For this review, take the finished solid that the model builds, in its own axes (mm). Face numbers are marked on the shaded views. A direction names the side the tool comes from. Coordinates: 2 decimals unless noted, no trailing zeros. Loops run counter-clockwise (first coordinate to the right, second up) from the corner with the lowest first, then second, coordinate; pieces in that order, holes last. Notation, with made-up numbers: (72, -10) -> (116, -10) arc R21 cw to (116, 4) -> close; hole circle Ø6 at (37.5, 86). An arc over 180 degrees is marked (long way). Answer in a Markdown table with one row per item.
from build123d import *

# Parameters (mm, degrees)
SKETCH_1_R          = 1
EXTRUDE_1_DEPTH     = 2
SKETCH_2_W          = 41
SKETCH_2_H          = 25.9
EXTRUDE_2_DEPTH     = 9.6
CUT_EXTRUDE_1_DEPTH = 49.428323324
CUT_EXTRUDE_2_DEPTH = 0.7
SKETCH_5_R          = 1.25
EXTRUDE_3_DEPTH     = 2
SKETCH_6_R          = 4
EXTRUDE_4_DEPTH     = 4
EXTRUDE_4_TAPER     = 10
SKETCH_7_R          = 2.1
EXTRUDE_5_DEPTH     = 2
SKETCH_8_W          = 12
SKETCH_8_H          = 4.5
CUT_EXTRUDE_3_DEPTH = 0.5
SKETCH_9_W          = 7
SKETCH_9_H          = 4.2
SKETCH_9_W_2        = 6
CUT_EXTRUDE_4_DEPTH = 0.5
SKETCH_12_W         = 3
SKETCH_12_H         = 1
CUT_EXTRUDE_5_DEPTH = 0.5
SKETCH_13_W         = 1.5
SKETCH_13_H         = 1
EXTRUDE_6_DEPTH     = 1


with BuildPart() as part:
    # 草图1 → 凸台-拉伸1 (new body)
    with BuildSketch(Plane(origin=(0, 0, 0), x_dir=(1, 0, 0), z_dir=(0, 1, 0))):
        Polygon((-20.75, 12.95), (20.75, 12.95), (24.7, 9.5), (24.7, -9.5), (20.75, -12.95), (-20.75, -12.95), (-24.7, -9.5), (-24.7, 9.5), align=None)
        with Locations(Location((22.5, 9, 0), (0, 0, 270))):
            Circle(SKETCH_1_R, mode=Mode.SUBTRACT)
        with Locations(Location((22.5, -9, 0), (0, 0, 270))):
            Circle(SKETCH_1_R, mode=Mode.SUBTRACT)
        with Locations(Location((-22.5, -9, 0), (0, 0, 270))):
            Circle(SKETCH_1_R, mode=Mode.SUBTRACT)
        with Locations(Location((-22.5, 9, 0), (0, 0, 270))):
            Circle(SKETCH_1_R, mode=Mode.SUBTRACT)
    extrude(amount=EXTRUDE_1_DEPTH)

    # 草图2 → 凸台-拉伸2 (add)
    with BuildSketch(Plane(origin=(0, 2, 0), x_dir=(1, 0, 0), z_dir=(0, 1, 0))):
        Rectangle(SKETCH_2_W, SKETCH_2_H)
    extrude(amount=EXTRUDE_2_DEPTH)

    # 草图3 → 切除-拉伸1 (cut, through all)
    with BuildSketch(Plane(origin=(20.5, 0, 0), x_dir=(0, 0, -1), z_dir=(1, 0, 0))):
        Polygon((-5.5, 11.6), (-12.95, 10.9), (-12.95, 11.6), align=None)
        Polygon((12.95, 11.6), (5.5, 11.6), (12.95, 10.9), align=None)
    extrude(amount=-CUT_EXTRUDE_1_DEPTH, mode=Mode.SUBTRACT)

    # 草图4 → 切除-拉伸2 (cut)
    with BuildSketch(Plane(origin=(0, 11.6, 0), x_dir=(1, 0, 0), z_dir=(0, 1, 0))):
        Polygon((7.476685986, 12.95), (0, 0), (7.476685986, -12.95), (5.167284909, -12.95), (-2.309401077, 0), (5.167284909, 12.95), align=None)
        Polygon((2.857883832, 12.95), (-1.443375673, 5.5), (-10.840856662, 5.5), (-15.142116168, 12.95), align=None)
        Polygon((-1.443375673, -5.5), (2.857883832, -12.95), (-15.142116168, -12.95), (-10.840856662, -5.5), align=None)
    extrude(amount=-CUT_EXTRUDE_2_DEPTH, mode=Mode.SUBTRACT)

    # 草图5 → 凸台-拉伸3 (add)
    with BuildSketch(Plane.ZY.offset(20.5)):
        with Locations(Location((0, 3.5, 0), (0, 0, 180))):
            Circle(SKETCH_5_R)
        with Locations(Location((4, 3.5, 0), (0, 0, 180))):
            Circle(SKETCH_5_R)
        with Locations(Location((-4, 3.5, 0), (0, 0, 180))):
            Circle(SKETCH_5_R)
    extrude(amount=EXTRUDE_3_DEPTH)

    # 草图6 → 凸台-拉伸4 (add)
    with BuildSketch(Plane(origin=(20.5, 0, 0), x_dir=(0, 0, -1), z_dir=(1, 0, 0))):
        with Locations((0, 6.3)):
            Circle(SKETCH_6_R)
    extrude(amount=EXTRUDE_4_DEPTH, taper=EXTRUDE_4_TAPER)

    # 草图7 → 凸台-拉伸5 (add)
    with BuildSketch(Plane(origin=(24.5, 0, 0), x_dir=(0, 0, -1), z_dir=(1, 0, 0))):
        with Locations((0, 6.3)):
            Circle(SKETCH_7_R)
    extrude(amount=EXTRUDE_5_DEPTH)

    # 草图8 → 切除-拉伸3 (cut)
    with BuildSketch(Plane.ZY.offset(20.5)):
        with Locations((0, 8.25)):
            Rectangle(SKETCH_8_W, SKETCH_8_H)
    extrude(amount=-CUT_EXTRUDE_3_DEPTH, mode=Mode.SUBTRACT)

    # 草图9 → 切除-拉伸4 (cut)
    with BuildSketch(Plane(origin=(20.5, 0, 0), x_dir=(0, 0, -1), z_dir=(1, 0, 0))):
        with Locations((8.25, 8.1)):
            Rectangle(SKETCH_9_W, SKETCH_9_H)
        with Locations((-8.75, 8.1)):
            Rectangle(SKETCH_9_W_2, SKETCH_9_H)
    extrude(amount=-CUT_EXTRUDE_4_DEPTH, mode=Mode.SUBTRACT)

    # 草图12 → 切除-拉伸5 (cut)
    with BuildSketch(Plane.XY.offset(12.95)):
        with Locations((-0.5, 6.5)):
            Rectangle(SKETCH_12_W, SKETCH_12_H)
    extrude(amount=-CUT_EXTRUDE_5_DEPTH, mode=Mode.SUBTRACT)

    # 草图13 → 凸台-拉伸6 (add)
    with BuildSketch(Plane.XY.offset(12.45)):
        with Locations((0.25, 6.5)):
            Rectangle(SKETCH_13_W, SKETCH_13_H)
    extrude(amount=EXTRUDE_6_DEPTH)


solid = part.part
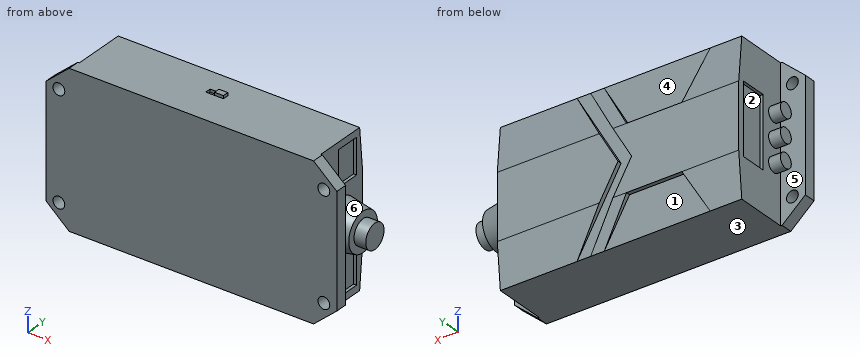
Item 1: For the marked faces 1, 2 and 3, list the 3-axis set-ups (+Z, -Z, +X, -X, +Y, -Y) from which the entire face can be reached by the end or side of a thin tool; tool diameter is ignored.
Worked answers:
| item | result |
|---|---|
| face 1 | -Z, +Y |
| face 2 | -X |
| face 3 | -Z, +X, -X, +Y, -Y |
Item 2: Take a section at C-C, the plane x = -11.5. State the section outline as (y, z) points.
Worked answers:
| item | result |
|---|---|
| outline | (0, -12.95) -> (10.9, -12.95) -> (10.9, -6.64) -> (11.49, -6.64) -> (11.6, -5.5) -> (11.6, 5.5) -> (11.49, 6.64) -> (10.9, 6.64) -> (10.9, 12.95) -> (0, 12.95) -> close |
Item 3: The part is to be moulded in two halves that separate along X. For the marked faces 4, 5 and 6, say which applies: +X half, -X half, draft (parallel to the pull), parting line (faces both ways), or undercut.
Worked answers:
| item | result |
|---|---|
| face 4 | undercut |
| face 5 | draft |
| face 6 | +X half |
Item 4: Take a section at A-A, the plane z = 9. State the section outline as (x, y) points, and give its area (3 significant figures).
Worked answers:
| item | result |
|---|---|
| outline | (-24.7, 0) -> (-23.5, 0) -> (-23.5, 2) -> (-24.7, 2) -> close; (-21.5, 0) -> (21.5, 0) -> (21.5, 2) -> (20.5, 2) -> (20.5, 6) -> (20, 6) -> (20, 10.2) -> (20.5, 10.2) -> (20.5, 11.27) -> (5.2, 11.27) -> (5.2, 10.9) -> (2.89, 10.9) -> (2.89, 11.27) -> (0.58, 11.27) -> (0.58, 10.9) -> (-12.86, 10.9) -> (-12.86, 11.27) -> (-20.5, 11.27) -> (-20.5, 2) -> (-21.5, 2) -> close; (23.5, 0) -> (24.7, 0) -> (24.7, 2) -> (23.5, 2) -> close |
| area | 463 mm² |
Item 5: Take a section at D-D, the plane z = -7. State the section outline as (x, y) points, and give its area (3 significant figures).
Worked answers:
| item | result |
|---|---|
| outline | (-24.7, 0) -> (24.7, 0) -> (24.7, 2) -> (20.5, 2) -> (20.5, 6) -> (20, 6) -> (20, 10.2) -> (20.5, 10.2) -> (20.5, 11.46) -> (4.04, 11.46) -> (4.04, 10.9) -> (1.73, 10.9) -> (1.73, 11.46) -> (-0.58, 11.46) -> (-0.58, 10.9) -> (-11.71, 10.9) -> (-11.71, 11.46) -> (-20.5, 11.46) -> (-20.5, 2) -> (-24.7, 2) -> close |
| area | 477 mm² |
Item 6: Insertion check: pin 1 (3 mm diameter, centred on y = 8, z = -6, fed in from -X); pin 2 (6 mm diameter, centred on x = 15.5, z = 10, fed in from +Y); pin 3 (1.2 mm diameter, centred on y = 3.5, z = -4, fed in from -X). Each pin has a flat end and moves straight along its axis. Give the tip position at first contact, or say it passes through.
Worked answers:
| item | result |
|---|---|
| pin 1 | x = -20.5 |
| pin 2 | y = 11.46 |
| pin 3 | x = -22.5 |
Item 7: Take a section at B-B, the plane x = 22.5. State the section outline as (y, z) points.
Worked answers:
| item | result |
|---|---|
| outline | (0, -11.42) -> (2, -11.42) -> (2, -10) -> (0, -10) -> close; (0, -8) -> (2, -8) -> (2, 8) -> (0, 8) -> close; (0, 10) -> (2, 10) -> (2, 11.42) -> (0, 11.42) -> close; circle Ø7.29 at (6.3, 0) |
Item 8: For L1, parallel to X at y = 1.1, z = 9; L2, parallel to Y at x = -13.5, z = 10.5; L3, parallel to X at y = 3, z = 11, list the stretches that pass through material, from the lowest coordinate up.
Worked answers:
| item | result |
|---|---|
| L1 | -24.7 to -23.5, -21.5 to 21.5, 23.5 to 24.7 |
| L2 | 0 to 10.9 |
| L3 | -20.5 to 20.5 |
